For this review, take the finished solid that the model builds, in its own axes (mm). Coordinates: 2 decimals unless noted, no trailing zeros. Order: outer loops, then holes, each group sorted by start corner. A loop starts at its lowest first (then second) coordinate and runs counter-clockwise, first axis right, second up.
from build123d import *

# Parameters (mm, degrees)
MODEL_R             = 0.4191
MODEL_R_2           = 0.227
MODEL_R_3           = 0.482663622
MODEL_R_4           = 0.43815
MODEL_R_5           = 0.9271
MODEL_R_6           = 0.425
MODEL_R_7           = 0.45
MODEL_R_8           = 1.524
MODEL_R_9           = 1.55
MODEL_R_10          = 1
MODEL_W             = 3.937
MODEL_H             = 23.478
BOSS_EXTRUDE1_DEPTH = 1.6129


with BuildPart() as part:
    # Model → Boss-Extrude1 (new body)
    with BuildSketch(Plane.XY):
        with BuildLine():
            Line((-23.779710926, -18.809832125), (-23.779710926, -17.398832125))
            ThreePointArc((-23.779710926, -17.398832125), (-24.125617817, -16.563739016), (-24.960710926, -16.217832125))
            ThreePointArc((-24.960710926, -16.217832125), (-27.082031269, -15.339152468), (-27.960710926, -13.217832125))
            ThreePointArc((-27.960710926, -13.217832125), (-27.082031269, -11.096511781), (-24.960710926, -10.217832125))
            ThreePointArc((-24.960710926, -10.217832125), (-24.253604145, -9.924938906), (-23.960710926, -9.217832125))
            Line((-23.960710926, -9.217832125), (-23.960710926, 14.782167875))
            ThreePointArc((-23.960710926, 14.782167875), (-24.253604145, 15.489274656), (-24.960710926, 15.782167875))
            ThreePointArc((-24.960710926, 15.782167875), (-27.082031269, 16.660847532), (-27.960710926, 18.782167875))
            ThreePointArc((-27.960710926, 18.782167875), (-27.082031269, 20.903488219), (-24.960710926, 21.782167875))
            ThreePointArc((-24.960710926, 21.782167875), (-24.253604145, 22.075061094), (-23.960710926, 22.782167875))
            Line((-23.960710926, 22.782167875), (-23.960710926, 25.782167875))
            ThreePointArc((-23.960710926, 25.782167875), (-15.463875449, 31.618102481), (-5.640710926, 34.742167875))
            Line((-5.640710926, 34.742167875), (-5.560710926, 34.742167875))
            ThreePointArc((-5.560710926, 34.742167875), (-4.86774628, 35.02920323), (-4.580710926, 35.722167875))
            ThreePointArc((-4.580710926, 35.722167875), (-4.369827808, 36.231284758), (-3.860710926, 36.442167875))
            Line((-3.860710926, 36.442167875), (4.609289074, 36.442167875))
            ThreePointArc((4.609289074, 36.442167875), (5.118407802, 36.231286158), (5.32929232, 35.72216859))
            ThreePointArc((5.32929232, 35.72216859), (5.651326218, 35.014708556), (6.379288359, 34.742171121))
            ThreePointArc((6.379288359, 34.742171121), (16.019672961, 31.575717146), (24.329289074, 25.752167875))
            Line((24.329289074, 25.752167875), (24.326289074, 22.516167875))
            ThreePointArc((24.326289074, 22.516167875), (24.619182293, 21.809061094), (25.326289074, 21.516167875))
            ThreePointArc((25.326289074, 21.516167875), (27.447609418, 20.637488219), (28.326289074, 18.516167875))
            ThreePointArc((28.326289074, 18.516167875), (27.447609418, 16.394847532), (25.326289074, 15.516167875))
            ThreePointArc((25.326289074, 15.516167875), (24.619182293, 15.223274656), (24.326289074, 14.516167875))
            Line((24.326289074, 14.516167875), (24.326289074, -9.483832125))
            ThreePointArc((24.326289074, -9.483832125), (24.619182293, -10.190938906), (25.326289074, -10.483832125))
            ThreePointArc((25.326289074, -10.483832125), (27.447609418, -11.362511781), (28.326289074, -13.483832125))
            ThreePointArc((28.326289074, -13.483832125), (27.447609418, -15.605152468), (25.326289074, -16.483832125))
            ThreePointArc((25.326289074, -16.483832125), (24.491195966, -16.829739016), (24.145289074, -17.664832125))
            Line((24.145289074, -17.664832125), (24.146689074, -19.076432125))
            ThreePointArc((24.146689074, -19.076432125), (0.126168598, -29.247573474), (-23.779710926, -18.809832125))
        make_face()
        with Locations((-3.370710926, -16.372832125)):
            Circle(MODEL_R, mode=Mode.SUBTRACT)
        with Locations((-0.830710926, -16.372832125)):
            Circle(MODEL_R, mode=Mode.SUBTRACT)
        with Locations((1.709289074, -16.372832125)):
            Circle(MODEL_R, mode=Mode.SUBTRACT)
        with Locations((4.249289074, -16.372832125)):
            Circle(MODEL_R, mode=Mode.SUBTRACT)
        with Locations((4.312789074, 7.804667875)):
            Circle(MODEL_R, mode=Mode.SUBTRACT)
        with Locations((1.772789074, 7.804667875)):
            Circle(MODEL_R, mode=Mode.SUBTRACT)
        with Locations((-0.767210926, 7.804667875)):
            Circle(MODEL_R, mode=Mode.SUBTRACT)
        with Locations((-3.307210926, 7.804667875)):
            Circle(MODEL_R, mode=Mode.SUBTRACT)
        with Locations((0.530089074, 13.311767875)):
            Circle(MODEL_R_2, mode=Mode.SUBTRACT)
        with Locations((-0.119910926, 14.311767875)):
            Circle(MODEL_R_2, mode=Mode.SUBTRACT)
        with Locations((1.830089074, 13.311767875)):
            Circle(MODEL_R_2, mode=Mode.SUBTRACT)
        with Locations((1.180089074, 14.311767875)):
            Circle(MODEL_R_2, mode=Mode.SUBTRACT)
        with Locations((-0.769910926, 13.311767875)):
            Circle(MODEL_R_2, mode=Mode.SUBTRACT)
        with Locations((14.214989074, 28.432167875)):
            Circle(MODEL_R_3, mode=Mode.SUBTRACT)
        with Locations((-20.168710926, 22.918167875)):
            Circle(MODEL_R_4, mode=Mode.SUBTRACT)
        with Locations((17.107289074, 26.303367875)):
            Circle(MODEL_R_3, mode=Mode.SUBTRACT)
        with Locations((-18.776910926, 20.064467875)):
            Circle(MODEL_R_4, mode=Mode.SUBTRACT)
        with Locations((-6.014510926, 29.821667875)):
            Circle(MODEL_R_4, mode=Mode.SUBTRACT)
        with Locations((-4.622710926, 26.967967875)):
            Circle(MODEL_R_4, mode=Mode.SUBTRACT)
        with Locations((-16.619110926, 22.883167875)):
            Circle(MODEL_R_5, mode=Mode.SUBTRACT)
        with Locations((-12.395710926, 24.943067875)):
            Circle(MODEL_R_5, mode=Mode.SUBTRACT)
        with Locations((-8.172210926, 27.002967875)):
            Circle(MODEL_R_5, mode=Mode.SUBTRACT)
        with Locations((2.339289074, 32.852167875)):
            Circle(MODEL_R_6, mode=Mode.SUBTRACT)
        with Locations((-1.460710926, 32.852167875)):
            Circle(MODEL_R_6, mode=Mode.SUBTRACT)
        with Locations((21.409289074, 21.770167875)):
            Circle(MODEL_R_7, mode=Mode.SUBTRACT)
        with Locations((21.409289074, 18.734167875)):
            Circle(MODEL_R_7, mode=Mode.SUBTRACT)
        with Locations((0.419289074, 27.993767875)):
            Circle(MODEL_R_8, mode=Mode.SUBTRACT)
        with Locations((-25.280710926, 18.783767875)):
            Circle(MODEL_R_9, mode=Mode.SUBTRACT)
        with Locations((-25.300710926, -13.226232125)):
            Circle(MODEL_R_9, mode=Mode.SUBTRACT)
        with Locations((0.439289074, -26.316232125)):
            Circle(MODEL_R_8, mode=Mode.SUBTRACT)
        with Locations((25.629289074, -13.486232125)):
            Circle(MODEL_R_9, mode=Mode.SUBTRACT)
        with Locations((25.659289074, 18.523767875)):
            Circle(MODEL_R_9, mode=Mode.SUBTRACT)
        with Locations((12.982089074, -16.238232125)):
            Circle(MODEL_R_10, mode=Mode.SUBTRACT)
        with BuildLine():
            Line((-2.85875692, 14.001767875), (-2.85875692, 13.216767875))
            ThreePointArc((-2.85875692, 13.216767875), (-3.038660926, 13.03686387), (-3.218564931, 13.216767875))
            Line((-3.218564931, 13.216767875), (-3.218564931, 14.001767875))
            ThreePointArc((-3.218564931, 14.001767875), (-3.038660926, 14.181671881), (-2.85875692, 14.001767875))
        make_face(mode=Mode.SUBTRACT)
        with BuildLine():
            Line((4.29124308, 14.001767875), (4.29124308, 13.216767875))
            ThreePointArc((4.29124308, 13.216767875), (4.111339074, 13.03686387), (3.931435069, 13.216767875))
            Line((3.931435069, 13.216767875), (3.931435069, 14.001767875))
            ThreePointArc((3.931435069, 14.001767875), (4.111339074, 14.181671881), (4.29124308, 14.001767875))
        make_face(mode=Mode.SUBTRACT)
        Polygon((2.128389074, -6.674157085), (2.128389074, -7.021507165), (1.882964114, -7.266932125), (1.535614034, -7.266932125), (1.290189074, -7.021507165), (1.290189074, -6.674157085), (1.535614034, -6.428732125), (1.882964114, -6.428732125), align=None, mode=Mode.SUBTRACT)
        Polygon((-0.411610926, -6.674157085), (-0.411610926, -7.021507165), (-0.657035886, -7.266932125), (-1.004385966, -7.266932125), (-1.249810926, -7.021507165), (-1.249810926, -6.674157085), (-1.004385966, -6.428732125), (-0.657035886, -6.428732125), align=None, mode=Mode.SUBTRACT)
        with Locations((16.800789074, -5.252332125)):
            Rectangle(MODEL_W, MODEL_H, mode=Mode.SUBTRACT)
    extrude(amount=BOSS_EXTRUDE1_DEPTH)


solid = part.part
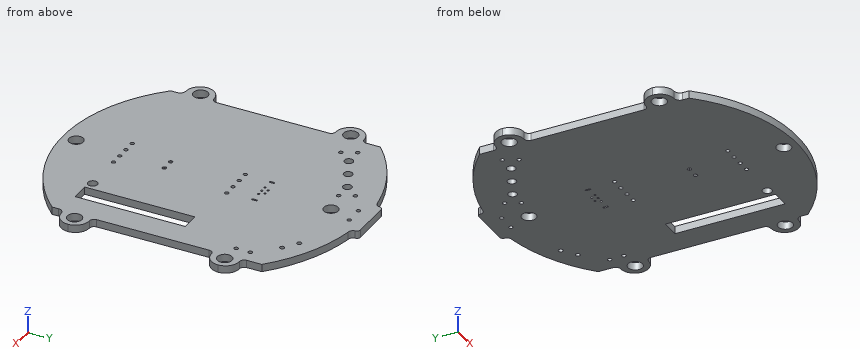
1. To check wall thickness, follow L1, parallel to X at y = -3.5, z = 0.55; L2, parallel to X at y = 13.5, z = 1.35; L3, parallel to Y at x = -4.5, z = 0.7. State the ranges of each line that lie inside material, in increasing order.
Answer below:
L1: x = -23.96 to 14.83, 18.77 to 24.33
L2: x = -23.96 to -3.22, -2.86 to -0.9, -0.64 to 0.4, 0.66 to 1.7, 1.96 to 3.93, 4.29 to 24.33
L3: y = -28.9 to 26.55, 27.39 to 36.05
2. Take a section at B-B, the plane z = 0.5. Give the number of separate pieces and of enclosed holes in the cut face, plus the area to 3 significant figures.
Answer below:
separate pieces: 1
enclosed holes: 38
area: 2,750 mm2
3. Clearance check with flat-ended pins moving along their axes: pin 1 Ø0.6 at (y, z) = (13.5, 1) entering from -X; pin 2 Ø0.8 at (x, z) = (17, 0.5) entering from -Y; pin 3 Ø0.6 at (y, z) = (14, 0.5) entering from +X. State where each tip first meets the part, or that it passes through.
Answer below:
pin 1: stops at x = -23.96
pin 2: stops at y = -24.95
pin 3: stops at x = 24.33
4. Take a section at A-A, the plane y = 0.5. Give the boundary of the cut face in (x, z), plus the area to 3 significant figures.
Answer below:
outline: (-23.96, 0) - (14.83, 0) - (14.83, 1.61) - (-23.96, 1.61) - close; (18.77, 0) - (24.33, 0) - (24.33, 1.61) - (18.77, 1.61) - close
area: 71.5 mm2
